from build123d import *

# Parameters (mm, degrees)
SKETCH1_W           = 35
SKETCH1_H           = 60
SKETCH1_R           = 6
SKETCH1_R_2         = 1.6
BOSS_EXTRUDE1_DEPTH = 10
SKETCH2_R           = 1.8
CUT_EXTRUDE1_DEPTH  = 10
CUT_EXTRUDE2_START  = -10
SKETCH3_R           = 1.8
CUT_EXTRUDE2_DEPTH  = 10
CUT_EXTRUDE3_DEPTH  = 5
FILLET1_R           = 6


with BuildPart() as part:
    # Sketch1 → Boss-Extrude1 (new body)
    with BuildSketch(Plane(origin=(0, 0, 0), x_dir=(0, 0, -1), z_dir=(1, 0, 0))):
        with Locations((17.5, 30)):
            Rectangle(SKETCH1_W, SKETCH1_H)
        with Locations((17.5, 51)):
            Circle(SKETCH1_R, mode=Mode.SUBTRACT)
        with Locations((6, 17)):
            Circle(SKETCH1_R_2, mode=Mode.SUBTRACT)
        with Locations((29, 17)):
            Circle(SKETCH1_R_2, mode=Mode.SUBTRACT)
    extrude(amount=BOSS_EXTRUDE1_DEPTH)

    # Sketch2 → Cut-Extrude1 (cut)
    with BuildSketch(Plane(origin=(0, 0, -35), x_dir=(-1, 0, 0), z_dir=(0, 0, -1))):
        with Locations((-5, 55)):
            Circle(SKETCH2_R)
        with Locations((-5, 30)):
            Circle(SKETCH2_R)
        with Locations((-5, 5)):
            Circle(SKETCH2_R)
    extrude(amount=-CUT_EXTRUDE1_DEPTH, mode=Mode.SUBTRACT)

    # Sketch3 → Cut-Extrude2 (cut)
    with BuildSketch(Plane.XY.offset(CUT_EXTRUDE2_START)):
        with Locations(Location((5, 55, 0), (0, 0, 180))):
            Circle(SKETCH3_R)
        with Locations(Location((5, 30, 0), (0, 0, 180))):
            Circle(SKETCH3_R)
        with Locations(Location((5, 5, 0), (0, 0, 180))):
            Circle(SKETCH3_R)
    extrude(amount=CUT_EXTRUDE2_DEPTH, mode=Mode.SUBTRACT)

    # Sketch4 → Cut-Extrude3 (cut)
    with BuildSketch(Plane(origin=(10, 0, 0), x_dir=(0, 0, -1), z_dir=(1, 0, 0))):
        with BuildLine():
            Line((29.5, 31.881008272), (29.5, 20.881008272))
            ThreePointArc((29.5, 20.881008272), (28.914213562, 19.466794709), (27.5, 18.881008272))
            Line((27.5, 18.881008272), (7.5, 18.881008272))
            ThreePointArc((7.5, 18.881008272), (6.085786438, 19.466794709), (5.5, 20.881008272))
            Line((5.5, 20.881008272), (5.5, 31.881008272))
            Line((5.5, 31.881008272), (5.5, 36.640158011))
            Line((5.5, 36.640158011), (5.5, 39.640158011))
            ThreePointArc((5.5, 39.640158011), (6.085786438, 41.054371573), (7.5, 41.640158011))
            Line((7.5, 41.640158011), (27.5, 41.640158011))
            ThreePointArc((27.5, 41.640158011), (28.914213562, 41.054371573), (29.5, 39.640158011))
            Line((29.5, 39.640158011), (29.5, 36.640158011))
            Line((29.5, 36.640158011), (29.5, 31.881008272))
        make_face()
    extrude(amount=-CUT_EXTRUDE3_DEPTH, mode=Mode.SUBTRACT)

    # Fillet1
    # the kernel refuses this fillet: 6 mm, written as the material it takes off along each edge
    with BuildSketch(Plane(origin=(0, 60, -50), x_dir=(0, -1, 0), z_dir=(0, 0, 1))) as fillet1_piece_1:
        with BuildLine():
            CenterArc((FILLET1_R, FILLET1_R), FILLET1_R, 180, 90)
            Line((0, FILLET1_R), (0, 0))
            Line((0, 0), (FILLET1_R, 0))
        make_face()
    extrude(amount=65, mode=Mode.SUBTRACT)
    with BuildSketch(Plane(origin=(0, 0, 15), x_dir=(1, 0, 0), z_dir=(0, 0, -1))) as fillet1_piece_2:
        with BuildLine():
            CenterArc((FILLET1_R, -FILLET1_R), FILLET1_R, 90, 90)
            Line((0, -FILLET1_R), (0, 0))
            Line((0, 0), (FILLET1_R, 0))
        make_face()
    extrude(amount=65, mode=Mode.SUBTRACT)


solid = part.part
Can you work these out from the model? Positions are in its coordinate system, mm. A direction names the side the tool comes from. Give positions to 0.01 mm unless a question says otherwise; leave off trailing zeros. Order: outer loops, then holes, each group sorted by start corner. A loop starts at its lowest first (then second) coordinate and runs counter-clockwise, first axis right, second up. Notation, with made-up numbers: M 78.25,16.25 L 101.25,16.25 A22 ccw 101.25,49.25 Z; hole C 54.5,39 d11. An arc over 180 degrees is marked long. One line per item, written item: value.
Item 1: If we mould it in two halves opening along Z, with no side actions, what happens to faces 4 (the face through (8, 0, -17)), 5 (the face through (8, 41.64, -17)), 6 (the face through (7, 30, -35))? For each: pulls with the +Z half, pulls with the -Z half, needs draft (parallel to the pull), parting line crosses it, or undercut.
Verdict:
face 4: needs draft
face 5: undercut
face 6: pulls with the -Z half
Item 2: Please list where these lines run through material, in increasing order: line 1 (Z direction, x = 9, y = 35.5); line 2 (Z direction, x = 4.25, y = 16.5); line 3 (Y direction, x = 4.25, z = -7).
Verdict:
line 1: -35 to -29.5, -5.5 to 0
line 2: -35 to -30.52, -27.48 to -7.52, -4.48 to 0
line 3: 0.26 to 3.36, 6.64 to 15.75, 18.25 to 28.36, 31.64 to 53.36, 56.64 to 59.74
Item 3: For pin 1 (3 mm diameter, centred on x = 5, y = 55, fed in from +Z); pin 2 (1.8 mm diameter, centred on x = 5.5, y = 55.5, fed in from -Z), each with a flat end and sliding along its axis, tell me the tip position at first contact or that it passes through.
Verdict:
pin 1: z = -10
pin 2: z = -25
Item 4: If we section it at D-D on x = 1.25: Write out the boundary of the cut face in (y, z).
Verdict:
outline: M 2.33,-35 L 57.67,-35 L 57.67,0 L 2.33,0 Z; hole C 17,-29 d3.2; hole C 17,-6 d3.2; hole C 51,-17.5 d12
Item 5: For faces 1 (the face through (8, 30, -29.5)), 2 (the face through (3.283, 55.541, -30.07)), 3 (the face through (3.283, 54.459, -5.07)), which set-ups out of +Z, -Z, +X, -X, +Y, -Y let a thin tool reach every point of the face, with its end or its side?
Verdict:
face 1: +X
face 2: -Z
face 3: +Z
Item 6: If we section it at A-A on y = 51: Write out the boundary of the cut face in (x, z), and give its area (3 significant figures).
Verdict:
outline: M 0,-35 L 10,-35 L 10,-23.5 L 0,-23.5 Z; M 0,-11.5 L 10,-11.5 L 10,0 L 0,0 Z
area: 230 mm2
Item 7: If we section it at C-C on z = -17.5: Write out the boundary of the cut face in (x, y).
Verdict:
outline: M 0,6 A6 ccw 6,0 L 10,0 L 10,18.88 L 5,18.88 L 5,41.64 L 10,41.64 L 10,45 L 0,45 Z; M 0.8,57 L 10,57 L 10,60 L 6,60 A6 ccw Z
Item 8: If we section it at B-B on x = 8.5: Write out the boundary of the cut face in (y, z), and give its area (3 significant figures).
Verdict:
outline: M 0,-35 L 60,-35 L 60,0 L 0,0 Z; hole C 17,-29 d3.2; hole C 17,-6 d3.2; hole M 18.88,-27.5 A2 ccw 20.88,-29.5 L 39.64,-29.5 A2 ccw 41.64,-27.5 L 41.64,-7.5 A2 ccw 39.64,-5.5 L 20.88,-5.5 A2 ccw 18.88,-7.5 Z; hole C 51,-17.5 d12
area: 1,430 mm2
